Drawing for the job (mm, zero at the part's lowest x, y, z). A direction names the side the tool comes from. Coordinates: 2 decimals unless noted, no trailing zeros. Loops run counter-clockwise (first coordinate to the right, second up) from the corner with the lowest first, then second, coordinate; pieces in that order, holes last. Notation, with made-up numbers: (47, -2.75) - (96, -2.75) arc R18 ccw to (96, 30.25) - close; hole circle Ø1 at (1, 24). An arc over 180 degrees is marked (long way). One line per item, written item: value.
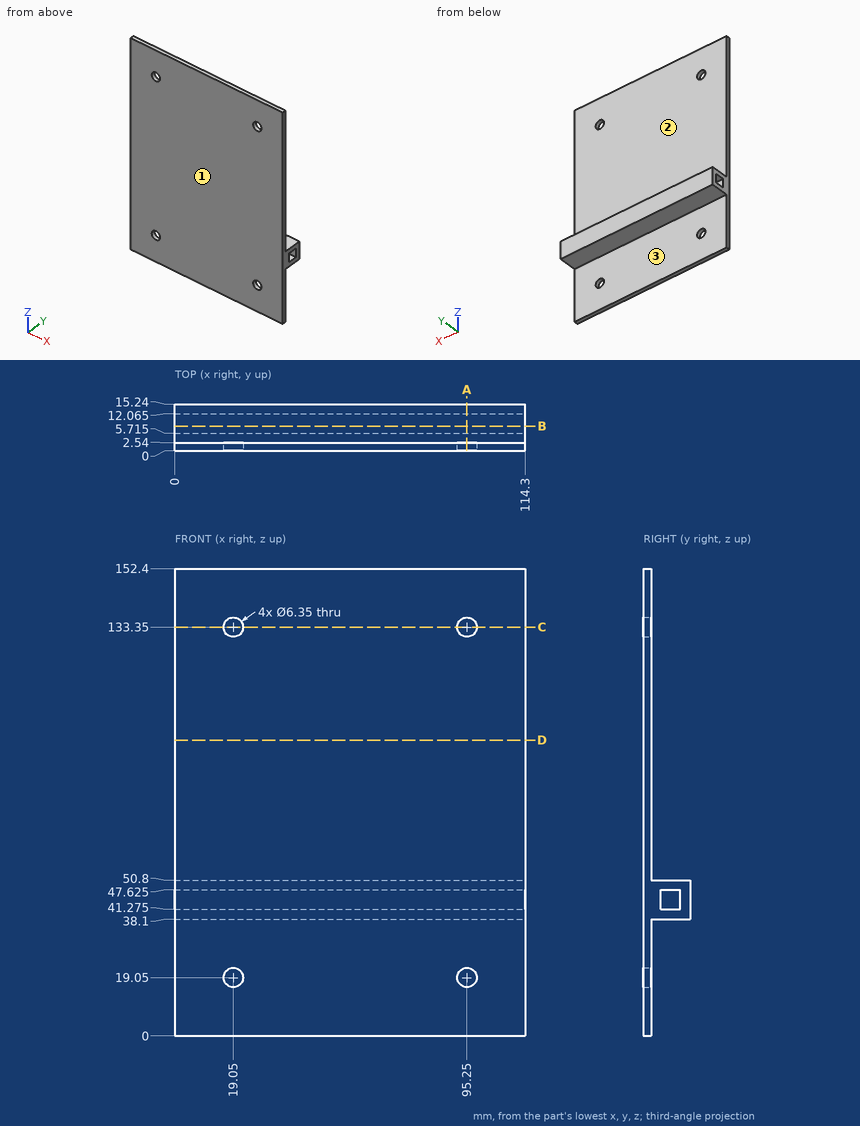
Item 1: Cut at D-D, the plane z = 96.5. Write the cut outline in (x, y), then the cut area to 3 significant figures.
Check result:
outline: (0, 0) - (114.3, 0) - (114.3, 2.54) - (0, 2.54) - close
area: 290 mm^2
Item 2: Probe probe 1 along Z at (x, y) = (95.25, 1.4) (3 decimals); probe 2 along X at (y, z) = (2.5, 19); probe 3 along Z at (x, y) = (21, 12) (3 decimals). List the from-to ranges inside material, lowest first. Write a range as from..to.
Check result:
probe 1: z = 0..15.875, 22.225..130.175, 136.525..152.4
probe 2: x = 0..15.88, 22.22..92.08, 98.42..114.3
probe 3: z = 38.1..41.275, 47.625..50.8
Item 3: Cut at A-A, the plane x = 95.25. Write the cut outline in (y, z) (3 decimals), then the cut area to 3 significant figures.
Check result:
outline: (0, 0) - (2.54, 0) - (2.54, 15.875) - (0, 15.875) - close; (0, 22.225) - (2.54, 22.225) - (2.54, 38.1) - (15.24, 38.1) - (15.24, 50.8) - (2.54, 50.8) - (2.54, 130.175) - (0, 130.175) - close; (0, 136.525) - (2.54, 136.525) - (2.54, 152.4) - (0, 152.4) - close; hole (5.715, 41.275) - (12.065, 41.275) - (12.065, 47.625) - (5.715, 47.625) - close
area: 476 mm^2
Item 4: Cut at C-C, the plane z = 133.35. Write the cut outline in (x, y) (3 decimals), then the cut area to 3 significant figures.
Check result:
outline: (0, 0) - (15.875, 0) - (15.875, 2.54) - (0, 2.54) - close; (22.225, 0) - (92.075, 0) - (92.075, 2.54) - (22.225, 2.54) - close; (98.425, 0) - (114.3, 0) - (114.3, 2.54) - (98.425, 2.54) - close
area: 258 mm^2
Item 5: Cut at B-B, the plane y = 8. Write the cut outline in (x, z) (3 decimals).
Check result:
outline: (0, 38.1) - (114.3, 38.1) - (114.3, 41.275) - (0, 41.275) - close; (0, 47.625) - (114.3, 47.625) - (114.3, 50.8) - (0, 50.8) - close
Item 6: Tool access for the marked faces 1, 2 and 3: list every direction of +Z, -Z, +X, -X, +Y, -Y with a clear straight run to the whole face (end or side of a thin tool).
Check result:
face 1: +Z, -Z, +X, -X, -Y
face 2: +Z, +X, -X, +Y
face 3: -Z, +X, -X, +Y
Item 7: Drop flat-ended pins along their axis: P1, Ø1.5, axis at x = 29.5, z = 59.5, coming from the +Y side; P2, Ø1.5, axis at x = 46.5, y = 4.5, coming from the +Z side; P3, Ø1.9, axis at x = 66, y = 9, coming from the -Z side. Give the stop position or say it passes through.
Check result:
P1: stops at y = 2.54
P2: stops at z = 50.8
P3: stops at z = 38.1
